Autodesk Inventor part; units mm, degrees
ref_plane "YZ Plane" through (0, 0, 0) normal (1, 0, 0) x (0, 1, 0)
ref_plane "XZ Plane" through (0, 0, 0) normal (0, 1, 0) x (-1, 0, 0)
ref_plane "XY Plane" through (0, 0, 0) normal (0, 0, 1) x (1, 0, 0)
sketch "Sketch2" plane through (0, 0, 0) normal (0, 0, 1) x (1, 0, 0)
  circle A0 centre (0, 0) radius 17.8
  dimension "d0" = 35.6
extrude "Extrusion1" add sketch "Sketch2" along normal blind 3
sketch "Sketch3" plane through (0, 0, 3) normal (0, 0, 1) x (1, 0, 0)
  circle A0 centre (0, 0) radius 6.5
  circle A1 centre (0, 0) radius 2
  arc A2 (-6.1065, 7.919) -> (-9.5399, 2.9985) centre (0, 0) ccw construction
  arc A3 (-7.3277, 9.5029) -> (-11.4478, 3.5982) centre (0, 0) ccw
  arc A4 (-4.8852, 6.3352) -> (-7.6319, 2.3988) centre (0, 0) ccw
  arc A5 (-4.8852, 6.3352) -> (-7.3277, 9.5029) centre (-6.1065, 7.919) ccw
  arc A6 (-11.4478, 3.5982) -> (-7.6319, 2.3988) centre (-9.5399, 2.9985) ccw
  circle A7 centre (0, 0) radius 17.8
  line L0 (0, 0) -> (-13.3383, 3.0709)
  line L1 (-16.7877, 5.9173) -> (-12.8896, 5.0199)
  line L2 (-12.8896, 5.0199) -> (-13.3383, 3.0709)
  line L3 (-17.6851, 2.0193) -> (-13.7871, 1.1219)
  line L4 (-13.7871, 1.1219) -> (-13.3383, 3.0709)
  arc A8 (-16.7877, 5.9173) -> (-17.6851, 2.0193) centre (0, 0) ccw
  arc A9 (-15.2021, 5.563) -> (-16.1032, 1.6551) centre (0, 0) ccw
  line L5 (-16.7877, 5.9173) -> (-15.2057, 5.5531)
  line L6 (-16.1032, 1.6551) -> (-17.6851, 2.0193)
  dimension "d3" = 13
  dimension "d4" = 4
  dimension "d18" = 10
  dimension "d20" = 4
  dimension "d26" = 4
  dimension "d27" = 2
  dimension "d33" = 6
extrude "Extrusion2" add sketch "Sketch3" along normal blind 3 contours A0
extrude "Extrusion3" cut sketch "Sketch3" against normal through all contours A1
extrude "Extrusion5" cut sketch "Sketch3" against normal blind 3 contours A6 L0 | L0 A6 A3 A5 A4
pattern_circular "Circular Pattern1" count 4 over 360 about axis through (0, 0, 3) along (0, 0, 1) of "Extrusion5"
extrude "Extrusion6" cut sketch "Sketch3" against normal blind 2 contours L4 L3 A9 L1 L2 | A9 L3 A7 L1
extrude "Extrusion7" cut sketch "Sketch3" against normal through all contours A9 L3 A7 L1
pattern_circular "Circular Pattern3" count 2 over 360 about axis through (0, 0, 3) along (0, 0, 1) of "Extrusion6", "Extrusion7"
properties part number "MotorFenek"
For this review, take the finished solid that the model builds, in its own axes (mm). A direction names the side the tool comes from. Round coordinates to 2 decimals unless told otherwise and drop trailing zeros. Order: outer loops, then holes, each group sorted by start corner. A loop starts at its lowest first (then second) coordinate and runs counter-clockwise, first axis right, second up. Notation, with made-up numbers: (25.5, 76.25) -> (68.5, 76.25) arc R32 ccw to (68.5, 105.25) -> close; hole circle Ø5 at (49.25, -13.75). An arc over 180 degrees is marked (long way). Write item = value, one per line. Start each with the question number.
1) The part is to be moulded in two halves that separate along Y. For faces 4 (the face through (-5.158, 3.955, 4.479)), 5 (the face through (0, -8, 3)), 6 (the face through (14.866, -5.475, 1.854)), say which applies: +Y half, -Y half, draft (parallel to the pull), parting line (faces both ways), or undercut.
2) To check wall thickness, follow line 1 (X direction, y = 0, z = 2.1); line 2 (Y direction, x = 0, z = 4.7). State the ranges of each line that lie inside material, in increasing order. Write a range as from..to.
3) Take a section at C-C on z = 2.25. State the section outline as (x, y) points.
4) Insertion check: pin 1 (10 mm diameter, centred on x = -9.5, y = 2, fed in from +Z); pin 2 (1.6 mm diameter, centred on x = -15, y = 3.5, fed in from +Z); pin 3 (1.5 mm diameter, centred on x = 7, z = 1.5, fed in from +Y); pin 4 (1.5 mm diameter, centred on x = 2, z = 3, fed in from +Y). Each pin has a flat end and moves straight along its axis. Give the tip position at first contact, or say it passes through.
5) Tool access review of faces 1 (the face through (-15, 3, 1)), 2 (the face through (-14.866, 5.475, 1.854)), 3 (the face through (6.54, -4.61, 1.52)): name each direction out of +Z, -Z, +X, -X, +Y, -Y from which nothing blocks a thin tool from reaching the whole face with its end or side.
6) Take a section at A-A on x = 0. State the section outline as (y, z) points.
Verdict:
q1.face_4 = parting line
q1.face_5 = draft
q1.face_6 = undercut
q2.line_1 = -17.8..-2, 2..17.8
q2.line_2 = -6.5..-2, 2..6.5
q3.outline = (-17.69, 2.02) arc R17.8 ccw to (16.79, -5.92) -> (12.89, -5.02) -> (13.34, -3.07) -> (13.79, -1.12) -> (17.69, -2.02) arc R17.8 ccw to (-16.79, 5.92) -> (-12.89, 5.02) -> (-13.34, 3.07) -> (-13.79, 1.12) -> close; hole (-11.45, 3.6) arc R2 ccw to (-7.63, 2.4) arc R8 cw to (-4.89, 6.34) arc R2 ccw to (-7.33, 9.5) arc R12 ccw to start; hole (-9.5, -7.33) arc R12 ccw to (-3.6, -11.45) arc R2 ccw to (-2.4, -7.63) arc R8 cw to (-6.34, -4.89) arc R2 ccw to start; hole circle Ø4 at (0, 0); hole (2.4, 7.63) arc R8 cw to (6.34, 4.89) arc R2 ccw to (9.5, 7.33) arc R12 ccw to (3.6, 11.45) arc R2 ccw to start; hole (4.89, -6.34) arc R2 ccw to (7.33, -9.5) arc R12 ccw to (11.45, -3.6) arc R2 ccw to (7.63, -2.4) arc R8 cw to start
q4.pin_1 = 6
q4.pin_2 = 1
q4.pin_3 = 16.67
q4.pin_4 = 17.76
q5.face_1 = +Z
q5.face_2 = +Z, -X
q5.face_3 = +Z, -Z
q6.outline = (-17.8, 0) -> (-2, 0) -> (-2, 6) -> (-6.5, 6) -> (-6.5, 3) -> (-17.8, 3) -> close; (2, 0) -> (17.8, 0) -> (17.8, 3) -> (6.5, 3) -> (6.5, 6) -> (2, 6) -> close
